Autodesk Inventor part; units mm, degrees
ref_plane "YZ Plane" through (0, 0, 0) normal (1, 0, 0) x (0, 1, 0)
ref_plane "XZ Plane" through (0, 0, 0) normal (0, 1, 0) x (-1, 0, 0)
ref_plane "XY Plane" through (0, 0, 0) normal (0, 0, 1) x (1, 0, 0)
ref_plane "Plan de construction1" through (0, 0, 0) normal (0, 0, 1) x (1, 0, 0)
sketch "Esquisse1" plane through (0, 0, 0) normal (0, 0, 1) x (1, 0, 0)
  arc A0 (39.951, -6.6629) -> (39.7815, -6.3404) centre (-6.5192, -30.8836) ccw
  arc A1 (37.1716, -5.7515) -> (36.5629, -4.7218) centre (-6.5192, -30.8836) ccw
  line L0 (-0.9849, 21.2268) -> (-0.9849, 19.2151)
  circle A2 centre (35, -6.3404) radius 2.25
  circle A3 centre (35, -6.3404) radius 2.25
  line L1 (32.8713, 2.0538) -> (-13.1447, 2.0538)
  line L2 (-13.1447, 2.0538) -> (-13.6192, -0.0461)
  line L3 (-13.6192, -0.0461) -> (30.4775, -0.0461)
  arc A4 (31.5995, 2.0932) -> (31.5733, 2.0538) centre (41.1898, -4.3006) ccw
  arc A5 (30.4775, -0.0461) -> (33.9606, -13.278) centre (41.1898, -4.3006) ccw
  arc A6 (39.7815, -6.3404) -> (32.8713, 2.0538) centre (19.4137, -16.066) ccw
  arc A7 (67.9818, -35.5103) -> (74.3699, -34.5283) centre (66.006, -1.387) ccw
  line L4 (74.3699, -28.9007) -> (74.3699, -34.5283)
  arc A8 (64.3223, -28.9007) -> (39.951, -6.6629) centre (33.5629, -38.1376) ccw
  arc A9 (57.8312, -28.9007) -> (33.9606, -13.278) centre (35.6884, -36.6859) ccw
  arc A10 (57.8312, -28.9007) -> (70.9309, -35.2107) centre (68.2954, -23.9295) ccw
  arc A11 (39.951, -6.6629) -> (39.977, -6.7609) centre (69.3461, 1.0787) ccw
  arc A12 (64.3223, -28.9007) -> (74.3699, -28.9007) centre (69.3461, 1.0787) ccw
  point P0 (0, 0)
  point P1 (32.8713, 3.678)
extrude "Extrusion1" add sketch "Esquisse1" along normal blind 4 contours A8 A12 L4 A7 A10 A9 A5 L3 L2 L1 A6 A0
ref_plane "Plan de construction2" through (0, 0, 13.25) normal (0, 0, 1) x (1, 0, 0)
mirror "Symétrie1" about plane through (0, 0, 13.25) normal (0, 0, 1) of "Extrusion1"
sketch "Esquisse4" plane through (0, 0, 4) normal (0, 0, 1) x (1, 0, 0)
  arc A0 (64.3223, -28.9007) -> (74.3699, -28.9007) centre (69.3461, 1.0787) ccw
  line L0 (74.3699, -34.5283) -> (74.3699, -28.9007)
  arc A1 (67.9818, -35.5103) -> (74.3699, -34.5283) centre (66.006, -1.387) ccw
  arc A2 (57.8312, -28.9007) -> (67.9818, -35.5103) centre (68.2954, -23.9295) ccw
  arc A3 (57.8312, -28.9007) -> (33.9606, -13.278) centre (35.6884, -36.6859) ccw
  arc A4 (64.3223, -28.9007) -> (39.951, -6.6629) centre (33.5629, -38.1376) ccw
  arc A5 (64.3223, -28.9007) -> (39.951, -6.6629) centre (33.5629, -38.1376) ccw
  line L1 (47.1623, -9.0426) -> (44.7261, -15.0241)
  arc A6 (57.8312, -28.9007) -> (33.9606, -13.278) centre (35.6884, -36.6859) ccw
  point P0 (0, 0)
extrude "Extrusion5" add sketch "Esquisse4" along normal blind 19.25
properties part number "courbe"
Part model, mm, in its own coordinate system. Round coordinates to 2 decimals unless told otherwise and drop trailing zeros. Order: outer loops, then holes, each group sorted by start corner. A loop starts at its lowest first (then second) coordinate and runs counter-clockwise, first axis right, second up. Notation, with made-up numbers: M -15.5,28.5 L 14.5,28.5 A35 cw 14.5,61.5 Z; hole C 9.5,-10.75 d3. An arc over 180 degrees is marked long. Put each result on its own line as item: value. Start each with the question number.
1. Slice it at A-A on x = 2. List the corners of the cut face in (y, z), then the cut area to 3 significant figures.
2. Drill centre lines: probe 1 along Y at (x, z) = (35, 23.7); probe 2 along X at (y, z) = (-10, 18.75); probe 3 along X at (y, z) = (-3, 2.25). Where is each one in solid material? Low to high. Write a range as [from, to].
3. Slice it at C-C on x = 35. List the corners of the cut face in (y, z).
4. Slice it at B-B on z = 9. List the corners of the cut face in (x, y).
5. Two-plate mould, pull along X, no slides. Class faces 1 (the face through (10, 2.054, 25)), 2 (the face through (36.89, -1.78, 24.53)), 3 (the face through (37.08, -7.2, 24.53)): +X half, -X half, draft (parallel to the pull), parting line (faces both ways), or undercut.
6. Slice it at D-D on y = -12. List the corners of the cut face in (x, z), then the cut area to 3 significant figures.
7. Drop flat-ended pins along their axis: pin 1 (12 mm diameter, centred on y = -30, z = 8.5, fed in from -X); pin 2 (1.2 mm diameter, centred on x = 14.5, z = 2, fed in from -Y); pin 3 (1 mm diameter, centred on x = 50, z = 15.5, fed in from -Y). Give the stop position or say it passes through.
Findings:
1. outline: M -0.05,0 L 2.05,0 L 2.05,4 L -0.05,4 Z; M -0.05,22.5 L 2.05,22.5 L 2.05,26.5 L -0.05,26.5 Z
1. area: 16.8 mm2
2. probe 1: [-13.22, -8.59], [-4.09, 0.26]
2. probe 2: [46.77, 49.05]
2. probe 3: [29.74, 37.82]
3. outline: M -13.22,0 L -8.59,0 L -8.59,4 L -13.22,4 Z; M -13.22,22.5 L -8.59,22.5 L -8.59,26.5 L -13.22,26.5 Z; M -4.09,0 L 0.26,0 L 0.26,4 L -4.09,4 Z; M -4.09,22.5 L 0.26,22.5 L 0.26,26.5 L -4.09,26.5 Z
4. outline: M 44.73,-15.02 A23.47 cw 57.83,-28.9 A11.59 ccw 67.98,-35.51 A34.18 ccw 74.37,-34.53 L 74.37,-28.9 A30.4 cw 64.32,-28.9 A32.12 ccw 47.16,-9.04 Z
5. face 1: draft
5. face 2: +X half
5. face 3: undercut
6. outline: M 32.61,0 L 52.23,0 L 52.23,26.5 L 32.61,26.5 L 32.61,22.5 L 45.96,22.5 L 45.96,4 L 32.61,4 Z
6. area: 273 mm2
7. pin 1: x = 55.44
7. pin 2: y = -0.05
7. pin 3: y = -18.48
